```python
from build123d import *

# Parameters (mm, degrees)
SKETCH2_W               = 3
SKETCH2_H               = 18.2
BOSS_EXTRUDE1_DEPTH     = 24
CIRPATTERN1_COUNT       = 6
CUT_EXTRUDE1_DEPTH      = 41.546269865
CUT_EXTRUDE1_DEPTH_BACK = 41.546269865
SKETCH3_W               = 4.3
SKETCH3_H               = 4.3
FILLET1_R               = 2
FILLET2_R               = 2


with BuildPart() as part:
    # Sketch1 → Revolve1 (revolve)
    with BuildSketch(Plane(origin=(0, 0, 0), x_dir=(0, 0, -1), z_dir=(1, 0, 0)), mode=Mode.PRIVATE) as revolve1_sk:
        Polygon((0, 22), (1.7, 22), (1.7, 20.2), (4.2, 20.2), (4.2, 22), (6.2, 22), (6.5, 20.2), (19.5, 20.2), (19.8, 22), (21.8, 22), (21.8, 20.2), (24.3, 20.2), (24.3, 22), (26, 22), (26, 18.2), (0, 18.2), align=None)
    revolve(revolve1_sk.sketch.rotate(Axis((0, 0, 0.322174052), (0, 0, -1)), 90), axis=Axis((0, 0, 0.322174052), (0, 0, -1)))

    # Sketch2 → Boss-Extrude1 (add)
    with BuildSketch(Plane.XY):
        with Locations((0, 9.1)):
            Rectangle(SKETCH2_W, SKETCH2_H)
    boss_extrude1 = extrude(amount=-BOSS_EXTRUDE1_DEPTH)

    # CirPattern1: Boss-Extrude1 ×6 about axis
    cirpattern1_axis = Axis((0, 0, 0), (0, 0, 1))
    for i in range(1, CIRPATTERN1_COUNT):
        add(boss_extrude1.rotate(cirpattern1_axis, i * 360 / CIRPATTERN1_COUNT))

    # Sketch3 → Cut-Extrude1 (cut, two sides: drawn at the far end of the back side and taken through both)
    with BuildSketch(Plane.XY.offset(-CUT_EXTRUDE1_DEPTH_BACK)):
        Rectangle(SKETCH3_W, SKETCH3_H)
    extrude(amount=CUT_EXTRUDE1_DEPTH + CUT_EXTRUDE1_DEPTH_BACK, mode=Mode.SUBTRACT)

    # Fillet1
    fillet1_edges = [part.edges().sort_by_distance(p)[0] for p in [
        (14.958039343, 10.368078849, -12),
        (-14.958039343, 10.368078849, -12),
        (-1.5, 18.138081486, -12),
        (1.5, 18.138081486, -12),
        (-16.458039343, 7.770002637, -12),
        (-14.958039343, -10.368078849, -12),
        (-16.458039343, -7.770002637, -12),
        (1.5, -18.138081486, -12),
        (-1.5, -18.138081486, -12),
        (14.958039343, -10.368078849, -12),
        (16.458039343, -7.770002637, -12),
        (16.458039343, 7.770002637, -12),
        (3, 0, -12),
        (1.5, -2.598076211, -12),
        (-1.5, -2.598076211, -12),
        (-3, 0, -12),
        (1.5, 2.598076211, -12),
        (-1.5, 2.598076211, -12),
    ]]
    fillet(fillet1_edges, radius=FILLET1_R)

    # Fillet2
    fillet2_edges = [part.edges().sort_by_distance(p)[0] for p in [
        (-18.2, 0, -26),
    ]]
    fillet(fillet2_edges, radius=FILLET2_R - 0.0001)  # a hair under: the kernel refuses the full size


solid = part.part
```
Design review of the part built by this model. Coordinates are the model's own, in mm. A direction names the side the tool comes from. Round coordinates to 2 decimals unless told otherwise and drop trailing zeros. Write item = value, one per line. Start each with the question number.
1) Clearance check with flat-ended pins moving along their axes: pin 1 (5 mm diameter, centred on y = 9, z = -9, fed in from +X); pin 2 (3 mm diameter, centred on y = -12, z = -6.5, fed in from -X); pin 3 (4 mm diameter, centred on x = -3.5, y = -4, fed in from -Z); pin 4 (12 mm diameter, centred on y = 0, z = -9.5, fed in from +X). State where each tip first meets the part, or that it passes through.
2) Wall thickness on probe 1 along Z at (x, y) = (9, -18.5); probe 2 along X at (y, z) = (-9.5, -11.5); probe 3 along Z at (x, y) = (12, -17.5): over which ranges is each line inside the solid? List them lowest first. Write a range as from..to.
3) Mouldability with a two-part tool opening along X and no side actions: class faces 1 (the face through (-10, 18, -4.2)), 2 (the face through (-4.769, 21.477, -5.214)), 3 (the face through (-1.5, 11, -12)) as +X half, -X half, draft (parallel to the pull), parting line (faces both ways), or undercut.
4) Take a section at A-A, the plane y = 0. Count the separate pieces of the cut face and the enclosed holes in it, plus the area to 3 significant figures.
5) Tool access review of faces 4 (the face through (-5, 0, -12)), 5 (the face through (9.32, 17.92, -23.07)): name each direction out of +Z, -Z, +X, -X, +Y, -Y from which nothing blocks a thin tool from reaching the whole face with its end or side.
Results list:
q1.pin_1 = 19.13
q1.pin_2 = -19.32
q1.pin_3 = -24
q1.pin_4 = 22
q2.probe_1 = -26..-24.3, -21.8..-19.56, -6.44..-4.2, -1.7..0
q2.probe_2 = -17.83..-13.34, -1.5..1.5, 13.34..17.83
q2.probe_3 = -26..-24.3, -21.8..-19.67, -6.33..-4.2, -1.7..0
q3.face_1 = draft
q3.face_2 = parting line
q3.face_3 = undercut
q4.separate_pieces = 4
q4.enclosed_holes = 0
q4.area = 267 mm²
q5.face_4 = +Z, -Z
q5.face_5 = none
